Input: part model. Units: mm. Frame: model coordinates. Face numbers are marked on the shaded views. Coordinates: 2 decimals unless noted, no trailing zeros. Loops run counter-clockwise (first coordinate to the right, second up) from the corner with the lowest first, then second, coordinate; pieces in that order, holes last.
Item 1: Contact query for a flat-ended pin moving along its axis: P1, Ø6.5, axis at x = 28.12, z = 9.36, coming from the -Y side. Output: stop coordinate, or through.
Item 2: Section B-B on x = 44. Return loops of the section in (y, z), and give its area (3 significant figures).
Item 3: Pull-direction query (Y, two-part tool) for the marked faces 1, 2 and 3; classes: released by +Y, released by -Y, zero draft, split by the parting line, or undercut.
Item 4: Section A-A on z = 19.25. Return loops of the section in (x, y), and give its area (3 significant figures).
Item 5: Section D-D on y = 7.5. Return loops of the section in (x, z).
Item 6: Ray query, line 1 along X through (y, z) = (9.75, 9.5); line 2 along X through (y, z) = (5.5, 1); line 3 along X through (y, z) = (8.25, 18.75). Return the intervals inside material, ascending.
Item 7: Section C-C on y = 1.5. Return loops of the section in (x, z), and give its area (3 significant figures).
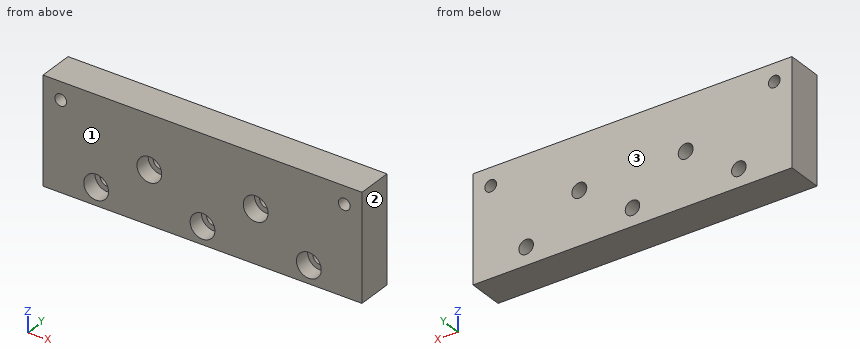
Autodesk Inventor part; units mm, degrees
ref_plane "YZ Plane" through (0, 0, 0) normal (1, 0, 0) x (0, 1, 0)
ref_plane "XZ Plane" through (0, 0, 0) normal (0, 1, 0) x (-1, 0, 0)
ref_plane "XY Plane" through (0, 0, 0) normal (0, 0, 1) x (1, 0, 0)
sketch "Sketch1" plane through (0, 0, 0) normal (0, 1, 0) x (-1, 0, 0)
  line L0 (31.8795, -5.6386) -> (-58.1205, -5.6386)
  line L1 (-58.1205, -5.6386) -> (-58.1205, 24.3614)
  line L2 (-58.1205, 24.3614) -> (31.8795, 24.3614)
  line L3 (31.8795, 24.3614) -> (31.8795, -5.6386)
  point P0 (0, 0)
  dimension "d0" = 90
  dimension "d5" = 30
extrude "Extrusion1" add sketch "Sketch1" along normal blind 10
sketch "Sketch2" plane through (0, 10, 0) normal (0, 1, 0) x (1, 0, 0)
  line L0 (58.1205, 5.6386) -> (-31.8795, 5.6386)
  line L1 (-31.8795, 5.6386) -> (-31.8795, -24.3614)
  circle A0 centre (-16.8795, 0.6386) radius 2.05
  circle A1 centre (13.1205, 0.6386) radius 2.05
  circle A2 centre (43.1205, 0.6386) radius 2.05
  point P0 (0, 0)
  dimension "d8" = 4.1
  dimension "d10" = 4.1
  dimension "d11" = 4.1
  dimension "d12" = 5
  dimension "d13" = 5
  dimension "d14" = 5
  dimension "d15" = 15
  dimension "d16" = 30
  dimension "d17" = 30
extrude "Extrusion2" cut sketch "Sketch2" against normal blind 10
sketch "Sketch4" plane through (0, 0, 0) normal (0, -1, 0) x (1, 0, 0)
  circle A0 centre (13.1205, -0.6386) radius 2.05
  circle A1 centre (-16.8795, -0.6386) radius 2.05
  circle A2 centre (43.1205, -0.6386) radius 2.05
  circle A3 centre (-16.8795, -0.6386) radius 3.5
  circle A4 centre (13.1205, -0.6386) radius 3.5
  circle A5 centre (43.1205, -0.6386) radius 3.5
  point P0 (0, 0)
  dimension "d26" = 7
  dimension "d28" = 7
  dimension "d29" = 7
extrude "Extrusion4" cut sketch "Sketch4" against normal blind 4.5
sketch "Sketch5" plane through (0, 0, 0) normal (0, -1, 0) x (1, 0, 0)
  line L0 (58.1205, -5.6386) -> (58.1205, 24.3614)
  line L1 (58.1205, 24.3614) -> (-31.8795, 24.3614)
  line L2 (-31.8795, 24.3614) -> (-31.8795, -5.6386)
  circle A0 centre (-1.8795, 9.3614) radius 2.1
  circle A1 centre (28.1205, 9.3614) radius 2.1
  point P0 (0, 0)
  dimension "d32" = 4.2
  dimension "d34" = 4.2
  dimension "d35" = 30
  dimension "d36" = 30
  dimension "d37" = 15
  dimension "d38" = 15
extrude "Extrusion5" cut sketch "Sketch5" against normal blind 10
sketch "Sketch6" plane through (0, 0, 0) normal (0, -1, 0) x (1, 0, 0)
  circle A0 centre (-1.8795, 9.3614) radius 2.1
  circle A1 centre (28.1205, 9.3614) radius 2.1
  circle A2 centre (-1.8795, 9.3614) radius 3.5
  circle A3 centre (28.1205, 9.3614) radius 3.5
  point P0 (0, 0)
  dimension "d41" = 7
  dimension "d43" = 7
extrude "Extrusion6" cut sketch "Sketch6" against normal blind 4.5
sketch "Sketch8" plane through (0, 10, 0) normal (0, 1, 0) x (1, 0, 0)
  line L0 (-31.8795, 5.6386) -> (-31.8795, -24.3614)
  line L1 (-31.8795, -24.3614) -> (-26.8795, -24.3614)
  line L2 (-26.8795, -24.3614) -> (-26.8795, -19.3614)
  line L3 (-26.8795, -19.3614) -> (-31.8795, -19.3614)
  line L4 (-31.8795, -19.3614) -> (-31.8795, -24.3614)
  line L5 (-31.8795, -24.3614) -> (58.1205, -24.3614)
  line L6 (58.1205, -24.3614) -> (53.1205, -24.3614)
  line L7 (53.1205, -24.3614) -> (53.1205, -19.3614)
  line L8 (53.1205, -19.3614) -> (58.1205, -19.3614)
  line L9 (58.1205, -19.3614) -> (58.1205, -24.3614)
  point P0 (0, 0)
  dimension "d58" = 5
  dimension "d59" = 5
  dimension "d62" = 5
  dimension "d63" = 5
hole "Hole1" at (-26.8795, 10, 19.3614) at (53.1205, 10, 19.3614) direction (0, -1, 0) diameter 3.302 depth 12.3
equation "\"d10\" = d8"
equation "\"d11\" = d8"
equation "\"d13\" = d12"
equation "\"d14\" = d12"
equation "\"d28\" = d26"
equation "\"d29\" = d26"
properties part number "AgarMouldBottomV3"
Results found:
1. P1: stops at y = 4.5
2. outline: (0, -5.64) - (10, -5.64) - (10, -2.49) - (4.5, -2.49) - (4.5, -4.03) - (0, -4.03) - close; (0, 2.75) - (4.5, 2.75) - (4.5, 1.21) - (10, 1.21) - (10, 24.36) - (0, 24.36) - close
2. area: 249 mm2
3. face 1: released by -Y
3. face 2: zero draft
3. face 3: released by +Y
4. outline: (-31.88, 0) - (-28.53, 0) - (-28.53, 10) - (-31.88, 10) - close; (-25.23, 0) - (51.47, 0) - (51.47, 10) - (-25.23, 10) - close; (54.77, 0) - (58.12, 0) - (58.12, 10) - (54.77, 10) - close
4. area: 834 mm2
5. outline: (-31.88, -5.64) - (58.12, -5.64) - (58.12, 24.36) - (-31.88, 24.36) - close; hole circle Ø3.3 at (-26.88, 19.36); hole circle Ø4.1 at (-16.88, -0.64); hole circle Ø4.2 at (-1.88, 9.36); hole circle Ø4.1 at (13.12, -0.64); hole circle Ø4.2 at (28.12, 9.36); hole circle Ø4.1 at (43.12, -0.64); hole circle Ø3.3 at (53.12, 19.36)
6. line 1: x = -31.88 to -3.97, 0.22 to 26.03, 30.22 to 58.12
6. line 2: x = -31.88 to -18.11, -15.65 to 11.89, 14.35 to 41.89, 44.35 to 58.12
6. line 3: x = -31.88 to -28.41, -25.35 to 51.59, 54.65 to 58.12
7. outline: (-31.88, -5.64) - (58.12, -5.64) - (58.12, 24.36) - (-31.88, 24.36) - close; hole circle Ø3.3 at (-26.88, 19.36); hole circle Ø7 at (-16.88, -0.64); hole circle Ø7 at (-1.88, 9.36); hole circle Ø7 at (13.12, -0.64); hole circle Ø7 at (28.12, 9.36); hole circle Ø7 at (43.12, -0.64); hole circle Ø3.3 at (53.12, 19.36)
7. area: 2,490 mm2
